from build123d import *

# Parameters (mm, degrees)
SKETCH_1_W          = 117
SKETCH_1_H          = 45
EXTRUDE_1_DEPTH     = 7
FILLET_1_R          = 2
SKETCH_2_W          = 108.5
SKETCH_2_H          = 35.5
CUT_EXTRUDE_1_DEPTH = 5
SKETCH_3_R          = 1.55
CUT_EXTRUDE_2_DEPTH = 64.067424238
SKETCH_6_W          = 15
SKETCH_6_H          = 15
EXTRUDE_2_DEPTH     = 14
SKETCH_7_R          = 4
CUT_EXTRUDE_3_DEPTH = 73.823416564
FILLET_2_R          = 4
SKETCH_8_W          = 5
SKETCH_8_H          = 15
CUT_EXTRUDE_4_DEPTH = 20
SKETCH_9_W          = 20
SKETCH_9_H          = 35.5
EXTRUDE_3_DEPTH     = 1.5


with BuildPart() as part:
    # 草图1 → 凸台-拉伸1 (new body)
    with BuildSketch(Plane.XY):
        Rectangle(SKETCH_1_W, SKETCH_1_H)
    extrude(amount=EXTRUDE_1_DEPTH)

    # 圆角1
    fillet_1_edges = [part.edges().sort_by_distance(p)[0] for p in [
        (58.5, -22.5, 3.5),
        (-58.5, -22.5, 3.5),
        (-58.5, 22.5, 3.5),
        (58.5, 22.5, 3.5),
    ]]
    fillet(fillet_1_edges, radius=FILLET_1_R)

    # 草图2 → 切除-拉伸1 (cut)
    with BuildSketch(Plane(origin=(0, 0, 0), x_dir=(-1, 0, 0), z_dir=(0, 0, -1))):
        Rectangle(SKETCH_2_W, SKETCH_2_H)
    extrude(amount=-CUT_EXTRUDE_1_DEPTH, mode=Mode.SUBTRACT)

    # 草图3 → 切除-拉伸2 (cut, through all)
    with BuildSketch(Plane(origin=(0, 0, 0), x_dir=(-1, 0, 0), z_dir=(0, 0, -1))):
        with Locations((-56.2, 20.2)):
            Circle(SKETCH_3_R)
        with Locations(Location((-56.2, -20.2, 0), (0, 0, 180))):
            Circle(SKETCH_3_R)
        with Locations((56.2, -20.2)):
            Circle(SKETCH_3_R)
        with Locations(Location((56.2, 20.2, 0), (0, 0, 180))):
            Circle(SKETCH_3_R)
    extrude(amount=-CUT_EXTRUDE_2_DEPTH, mode=Mode.SUBTRACT)

    # 草图6 → 凸台-拉伸2 (add)
    with BuildSketch(Plane.XY.offset(7)):
        Rectangle(SKETCH_6_W, SKETCH_6_H)
    extrude(amount=EXTRUDE_2_DEPTH)

    # 草图7 → 切除-拉伸3 (cut, through all)
    with BuildSketch(Plane.ZY.offset(7.5)):
        with Locations((15, 0)):
            Circle(SKETCH_7_R)
    extrude(amount=-CUT_EXTRUDE_3_DEPTH, mode=Mode.SUBTRACT)

    # 圆角2
    fillet_2_edges = [part.edges().sort_by_distance(p)[0] for p in [
        (0, -7.5, 21),
        (0, 7.5, 21),
    ]]
    fillet(fillet_2_edges, radius=FILLET_2_R)

    # 草图8 → 切除-拉伸4 (cut)
    with BuildSketch(Plane.XY.offset(7)):
        Rectangle(SKETCH_8_W, SKETCH_8_H)
    extrude(amount=CUT_EXTRUDE_4_DEPTH, mode=Mode.SUBTRACT)

    # 草图9 → 凸台-拉伸3 (add)
    with BuildSketch(Plane(origin=(0, 0, 5), x_dir=(-1, 0, 0), z_dir=(0, 0, -1))):
        with Locations((-44.25, 0)):
            Rectangle(SKETCH_9_W, SKETCH_9_H)
        with Locations((44.25, 0)):
            Rectangle(SKETCH_9_W, SKETCH_9_H)
    extrude(amount=EXTRUDE_3_DEPTH)


solid = part.part
Geometry: final body of the model. Coordinates: model frame, mm. A direction names the side the tool comes from. Coordinates: 2 decimals unless noted, no trailing zeros. Loops run counter-clockwise (first coordinate to the right, second up) from the corner with the lowest first, then second, coordinate; pieces in that order, holes last. Notation, with made-up numbers: (-23, 41) - (33, 41) arc R27 ccw to (33, 71) - close; hole circle Ø4 at (84, 13). An arc over 180 degrees is marked (long way). Put each result on its own line as item: value. Start each with the question number.
Q1. Pull-direction query (Y, two-part tool) for faces 5 (the flat face through (58.5, 0, 3)), 6 (the cylindrical face through (5.035, -6.359, 19.797)), 7 (the cylindrical face through (-55.37, 18.89, 3.45)); classes: released by +Y, released by -Y, zero draft, split by the parting line, or undercut.
Q2. Cut plane A-A, the plane y = 0. Return loops of the section in (x, z).
Q3. Set-up query: faces 1 (the flat face through (-7.5, -0.1, 10.8)), 2 (the flat face through (-54.25, 0, 2)), 3 (the flat face through (2.5, -0.1, 10.8)), 4 (the flat face through (-5, -7.5, 12)). Return all of +Z, -Z, +X, -X, +Y, -Y with unobstructed straight access to the full face (end or side cutting, diameter ignored); none if empty.
Q4. Cut plane D-D, the plane y = 14. Return loops of the section in (x, z).
Q5. Pin query (flat end, axial travel): pin 1 Ø18 at (x, y) = (-0.5, -7.5) entering from -Z; pin 2 Ø1 at (x, y) = (-39.5, -15) entering from -Z; pin 3 Ø5 at (x, y) = (56.2, 20.2) entering from +Z; pin 4 Ø6 at (x, y) = (-1, -0.5) entering from +Z. Return the tip coordinate at first contact, or that it passes through.
Q6. Line query: line 1 (Y direction, x = -56.2, z = 5.25); line 2 (X direction, y = -20, z = 6.5); line 3 (Z direction, x = 39.5, y = 7). Output: solid intervals per line, ascending.
Q7. Cut plane C-C, the plane x = -45.5. Return loops of the section in (y, z).
Q8. Cut plane B-B, the plane z = 15. Return loops of the section in (x, y), and give its area (3 significant figures).
Filled sheet:
1. face 5: zero draft
1. face 6: released by -Y
1. face 7: undercut
2. outline: (-58.5, 0) - (-54.25, 0) - (-54.25, 3.5) - (-34.25, 3.5) - (-34.25, 5) - (34.25, 5) - (34.25, 3.5) - (54.25, 3.5) - (54.25, 0) - (58.5, 0) - (58.5, 7) - (7.5, 7) - (7.5, 11) - (2.5, 11) - (2.5, 7) - (-2.5, 7) - (-2.5, 11) - (-7.5, 11) - (-7.5, 7) - (-58.5, 7) - close; (-7.5, 19) - (-2.5, 19) - (-2.5, 21) - (-7.5, 21) - close; (2.5, 19) - (7.5, 19) - (7.5, 21) - (2.5, 21) - close
3. face 1: +Z, -X, +Y, -Y
3. face 2: -Z
3. face 3: +Z, +Y, -Y
3. face 4: +Z, +X, -X, -Y
4. outline: (-58.5, 0) - (-54.25, 0) - (-54.25, 3.5) - (-34.25, 3.5) - (-34.25, 5) - (34.25, 5) - (34.25, 3.5) - (54.25, 3.5) - (54.25, 0) - (58.5, 0) - (58.5, 7) - (-58.5, 7) - close
5. pin 1: z = 5
5. pin 2: z = 3.5
5. pin 3: z = 7
5. pin 4: z = 21
6. line 1: -22.5 to -21.75, -18.65 to 18.65, 21.75 to 22.5
6. line 2: -58.5 to -57.74, -54.66 to 54.66, 57.74 to 58.5
6. line 3: 3.5 to 7
7. outline: (-22.5, 0) - (-17.75, 0) - (-17.75, 3.5) - (17.75, 3.5) - (17.75, 0) - (22.5, 0) - (22.5, 7) - (-22.5, 7) - close
8. outline: (-7.5, -7.5) - (-2.5, -7.5) - (-2.5, -4) - (-7.5, -4) - close; (-7.5, 4) - (-2.5, 4) - (-2.5, 7.5) - (-7.5, 7.5) - close; (2.5, -7.5) - (7.5, -7.5) - (7.5, -4) - (2.5, -4) - close; (2.5, 4) - (7.5, 4) - (7.5, 7.5) - (2.5, 7.5) - close
8. area: 70.0 mm²
